Autodesk Inventor part; units mm, degrees
ref_plane "YZ Plane" through (0, 0, 0) normal (1, 0, 0) x (0, 1, 0)
ref_plane "XZ Plane" through (0, 0, 0) normal (0, 1, 0) x (-1, 0, 0)
ref_plane "XY Plane" through (0, 0, 0) normal (0, 0, 1) x (1, 0, 0)
sketch "Sketch1" plane through (0, 0, 0) normal (0, 1, 0) x (-1, 0, 0)
  line L0 (3, 3) -> (-3, 3)
  line L1 (-3, 3) -> (-3, -3)
  line L2 (-3, -3) -> (3, -3)
  line L3 (3, -3) -> (3, 3)
  line L4 (3, 3) -> (-3, -3) construction
  line L5 (-3, 3) -> (3, -3) construction
  circle A0 centre (0, 0) radius 2
  point P0 (0, 0)
  dimension "d0" = 6
  dimension "d1" = 6
  dimension "d2" = 4
extrude "Extrusion1" add sketch "Sketch1" along normal blind 300
properties part number "carbon_fiber_200"
Design review of the part built by this model. Coordinates are the model's own, in mm. Round coordinates to 2 decimals unless told otherwise and drop trailing zeros. Order: outer loops, then holes, each group sorted by start corner. A loop starts at its lowest first (then second) coordinate and runs counter-clockwise, first axis right, second up. Notation, with made-up numbers: (48, 19) - (92, 19) arc R10 ccw to (92, 25) - close; hole circle Ø7 at (32.25, 49). An arc over 180 degrees is marked (long way). Return JSON: item names as keys, results as strings.
Q1. Consider section C-C on x = -0.6. Write out the cut boundary in (y, z).
Computed values:
{"outline": "(0, -3) - (300, -3) - (300, -1.91) - (0, -1.91) - close; (0, 1.91) - (300, 1.91) - (300, 3) - (0, 3) - close"}
Q2. Consider section A-A on z = 0. Write out the cut boundary in (x, y).
Computed values:
{"outline": "(-3, 0) - (-2, 0) - (-2, 300) - (-3, 300) - close; (2, 0) - (3, 0) - (3, 300) - (2, 300) - close"}
Q3. Wall thickness on L1, parallel to Z at x = 0, y = 209.5; L2, parallel to X at y = 67.5, z = 0.2; L3, parallel to Z at x = -0.45, y = 276.5: over which ranges is each line inside the solid? List them lowest first. Write a range as [from, to].
Computed values:
{"L1": "z = [-3, -2], [2, 3]", "L2": "x = [-3, -1.99], [1.99, 3]", "L3": "z = [-3, -1.95], [1.95, 3]"}
Q4. Consider section B-B on y = 194.5. Write out the cut boundary in (x, z), plus the area to 3 significant figures.
Computed values:
{"outline": "(-3, -3) - (3, -3) - (3, 3) - (-3, 3) - close; hole circle Ø4 at (0, 0)", "area": "23.4 mm2"}
